```python
from build123d import *

# Parameters (mm, degrees)
SKICA1_W                 = 96
SKICA1_H                 = 5
SKICA2_R                 = 3
ODEBRAT_VYSUNUT_M1_DEPTH = 5
ZAOBLIT1_R               = 1
SKICA3_R                 = 5.5
ODEBRAT_VYSUNUT_M2_DEPTH = 4
ZKOSEN_2_SIZE            = 0.5
SKICA4_R                 = 9
ODEBRAT_VYSUNUT_M3_DEPTH = 1.6
ZKOSEN_3_SIZE            = 0.5
SKICA5_W                 = 5
SKICA5_H                 = 5
P_IDAT_VYSUNUT_M1_DEPTH  = 10
ZKOSEN_8_SIZE            = 1
ODEBRAT_VYSUNUT_M4_DEPTH = 0.5


with BuildPart() as part:
    # Skica1 → Rotovat1 (revolve)
    with BuildSketch(Plane.XY, mode=Mode.PRIVATE) as rotovat1_sk:
        with Locations((-52, 2.5)):
            Rectangle(SKICA1_W, SKICA1_H)
    revolve(rotovat1_sk.sketch.rotate(Axis((0, 0, 0), (0, 1, 0)), 270), axis=Axis((0, 0, 0), (0, 1, 0)))

    # Skica2 → Odebrat vysunutím1 (cut)
    with BuildSketch(Plane(origin=(0, 5, 0), x_dir=(1, 0, 0), z_dir=(0, 1, 0))):
        with Locations(Location((0, 22.5, 0), (0, 0, 270))):
            Circle(SKICA2_R)
        with Locations(Location((21.398771617, 6.952882373, 0), (0, 0, 270))):
            Circle(SKICA2_R)
        with Locations(Location((13.225168177, -18.202882373, 0), (0, 0, 270))):
            Circle(SKICA2_R)
        with Locations(Location((-13.225168177, -18.202882373, 0), (0, 0, 270))):
            Circle(SKICA2_R)
        with Locations(Location((-21.398771617, 6.952882373, 0), (0, 0, 270))):
            Circle(SKICA2_R)
    extrude(amount=-ODEBRAT_VYSUNUT_M1_DEPTH, mode=Mode.SUBTRACT)

    # Zaoblit1
    zaoblit1_edges = [part.edges().sort_by_distance(p)[0] for p in [
        (0, 0, 100),
        (0, 5, 100),
    ]]
    fillet(zaoblit1_edges, radius=ZAOBLIT1_R)

    # Skica3 → Odebrat vysunutím2 (cut)
    with BuildSketch(Plane(origin=(0, 5, 0), x_dir=(1, 0, 0), z_dir=(0, 1, 0))):
        with Locations(Location((0, 22.5, 0), (0, 0, 270))):
            Circle(SKICA3_R)
        with Locations(Location((21.398771617, 6.952882373, 0), (0, 0, 270))):
            Circle(SKICA3_R)
        with Locations(Location((13.225168177, -18.202882373, 0), (0, 0, 270))):
            Circle(SKICA3_R)
        with Locations(Location((-13.225168177, -18.202882373, 0), (0, 0, 270))):
            Circle(SKICA3_R)
        with Locations(Location((-21.398771617, 6.952882373, 0), (0, 0, 270))):
            Circle(SKICA3_R)
    extrude(amount=-ODEBRAT_VYSUNUT_M2_DEPTH, mode=Mode.SUBTRACT)

    # Zkosení2
    zkosen_2_edges = [part.edges().sort_by_distance(p)[0] for p in [
        (0, 5, -28),
        (21.398771617, 5, -12.452882373),
        (13.225168177, 5, 12.702882373),
        (-13.225168177, 5, 12.702882373),
        (-21.398771617, 5, -12.452882373),
    ]]
    chamfer(zkosen_2_edges, length=ZKOSEN_2_SIZE)

    # Skica4 → Odebrat vysunutím3 (cut)
    with BuildSketch(Plane.XZ):
        with Locations(Location((0, 0, 0), (0, 0, 270))):
            Circle(SKICA4_R)
    extrude(amount=-ODEBRAT_VYSUNUT_M3_DEPTH, mode=Mode.SUBTRACT)

    # Zkosení3
    zkosen_3_edges = [part.edges().sort_by_distance(p)[0] for p in [
        (0, 5, 4),
    ]]
    chamfer(zkosen_3_edges, length=ZKOSEN_3_SIZE)

    # Skica5 → Přidat vysunutím1 (add)
    with BuildSketch(Plane.XZ):
        with Locations((-60, 0)):
            Rectangle(SKICA5_W, SKICA5_H)
    extrude(amount=P_IDAT_VYSUNUT_M1_DEPTH)

    # Zkosení8
    zkosen_8_edges = [part.edges().sort_by_distance(p)[0] for p in [
        (-57.5, 0, 0),
        (-60, 0, 2.5),
        (-62.5, 0, 0),
        (-60, 0, -2.5),
        (-57.5, -10, 0),
        (-60, -10, 2.5),
        (-62.5, -10, 0),
        (-60, -10, -2.5),
    ]]
    chamfer(zkosen_8_edges, length=ZKOSEN_8_SIZE)

    # Skica6 → Odebrat vysunutím4 (cut)
    with BuildSketch(Plane(origin=(0, 5, 0), x_dir=(1, 0, 0), z_dir=(0, 1, 0))):
        with BuildLine():
            Line((-104.877493729, 1), (-80, 1))
            ThreePointArc((-80, 1), (-79, 0), (-80, -1))
            Line((-80, -1), (-104.877493729, -1))
            ThreePointArc((-104.877493729, -1), (-105.877493729, 0), (-104.877493729, 1))
        make_face()
        with BuildLine():
            Line((-73.452480229, 74.866693791), (-55.861435714, 57.275649276))
            ThreePointArc((-55.861435714, 57.275649276), (-55.861435714, 55.861435714), (-57.275649276, 55.861435714))
            Line((-57.275649276, 55.861435714), (-74.866693791, 73.452480229))
            ThreePointArc((-74.866693791, 73.452480229), (-74.866693791, 74.866693791), (-73.452480229, 74.866693791))
        make_face()
        with BuildLine():
            Line((1, 104.877493729), (1, 80))
            ThreePointArc((1, 80), (0, 79), (-1, 80))
            Line((-1, 80), (-1, 104.877493729))
            ThreePointArc((-1, 104.877493729), (0, 105.877493729), (1, 104.877493729))
        make_face()
        with BuildLine():
            Line((74.866693791, 73.452480229), (57.275649276, 55.861435714))
            ThreePointArc((57.275649276, 55.861435714), (55.861435714, 55.861435714), (55.861435714, 57.275649276))
            Line((55.861435714, 57.275649276), (73.452480229, 74.866693791))
            ThreePointArc((73.452480229, 74.866693791), (74.866693791, 74.866693791), (74.866693791, 73.452480229))
        make_face()
        with BuildLine():
            Line((104.877493729, -1), (80, -1))
            ThreePointArc((80, -1), (79, 0), (80, 1))
            Line((80, 1), (104.877493729, 1))
            ThreePointArc((104.877493729, 1), (105.877493729, 0), (104.877493729, -1))
        make_face()
        with BuildLine():
            Line((73.452480229, -74.866693791), (55.861435714, -57.275649276))
            ThreePointArc((55.861435714, -57.275649276), (55.861435714, -55.861435714), (57.275649276, -55.861435714))
            Line((57.275649276, -55.861435714), (74.866693791, -73.452480229))
            ThreePointArc((74.866693791, -73.452480229), (74.866693791, -74.866693791), (73.452480229, -74.866693791))
        make_face()
        with BuildLine():
            Line((-1, -104.877493729), (-1, -80))
            ThreePointArc((-1, -80), (0, -79), (1, -80))
            Line((1, -80), (1, -104.877493729))
            ThreePointArc((1, -104.877493729), (0, -105.877493729), (-1, -104.877493729))
        make_face()
        with BuildLine():
            Line((-74.866693791, -73.452480229), (-57.275649276, -55.861435714))
            ThreePointArc((-57.275649276, -55.861435714), (-55.861435714, -55.861435714), (-55.861435714, -57.275649276))
            Line((-55.861435714, -57.275649276), (-73.452480229, -74.866693791))
            ThreePointArc((-73.452480229, -74.866693791), (-74.866693791, -74.866693791), (-74.866693791, -73.452480229))
        make_face()
    extrude(amount=-ODEBRAT_VYSUNUT_M4_DEPTH, mode=Mode.SUBTRACT)


solid = part.part
```
Can you work these out from the model? Positions are in its coordinate system, mm. A direction names the side the tool comes from. Coordinates: 2 decimals unless noted, no trailing zeros. Loops run counter-clockwise (first coordinate to the right, second up) from the corner with the lowest first, then second, coordinate; pieces in that order, holes last. Notation, with made-up numbers: (-13.75, 35) - (-8.75, 35) arc R32 cw to (-8.75, 61) - close; hole circle Ø2 at (-4.5, 89). An arc over 180 degrees is marked (long way). Answer as CSV lines item,"result". Start each with the question number.
1) I need wall thicknesses on line 1 (X direction, y = 3, z = 14.5); line 2 (Y direction, x = 8, z = 67); line 3 (X direction, y = 0.4, z = 0). Which ranges of each line are inside material? Lowest first, please. Write a range as from..to.
2) Thinking about a two-plate mould opening in Z: for faces 4 (the flat face through (63, 4.5, -63)), 5 (the flat face through (-62.5, -5, 0)), 6 (the flat face through (-60, -5, -2.5)), which applies, pulls with the +Z half, pulls with the -Z half, needs draft (parallel to the pull), parting line crosses it, or undercut?
3) For pin 1 (0.6 mm diameter, centred on x = 93.5, z = -0.5, fed in from +Y); pin 2 (4 mm diameter, centred on y = -4, z = 0.5, fed in from +X); pin 3 (4 mm diameter, centred on x = -59.5, y = -4.5, fed in from -Z), each with a flat end and sliding along its axis, tell me the tip position at first contact or that it passes through.
4) Suppose I cut it at A-A (y = -5.75). Please give me the cut outline in (x, z).
5) Suppose I cut it at B-B (z = 17.5). Count the separate pieces of the cut face and the enclosed holes in it, plus the area to 3 significant figures.
6) Which directions (+Z, -Z, +X, -X, +Y, -Y) give clear straight access to the entire face, cutting with the end or side of a thin tool? Please do faces 1 (the cylindrical face through (13.47, 2.77, 12.71)), 2 (the cylindrical face through (2.703, 0.789, -8.584)), 3 (the cylindrical face through (23.43, 0.51, -9.16)).
Check result:
1,line 1,"x = -98.94..-17.29, -9.16..9.16, 17.29..98.94"
1,line 2,"y = 0..5"
1,line 3,"x = -99.8..-9, 9..99.8"
2,face 4,"undercut"
2,face 5,"needs draft"
2,face 6,"pulls with the -Z half"
3,pin 1,"stops at y = 4.5"
3,pin 2,"stops at x = -57.5"
3,pin 3,"stops at z = -2.5"
4,outline,"(-62.5, -2.5) - (-57.5, -2.5) - (-57.5, 2.5) - (-62.5, 2.5) - close"
5,separate pieces,"3"
5,enclosed holes,"0"
5,area,"884 mm²"
6,face 1,"+Y"
6,face 2,"-Y"
6,face 3,"+Y, -Y"
